Input: part model. Units: mm. Frame: model coordinates. Face numbers are marked on the shaded views. A direction names the side the tool comes from. Give positions to 0.01 mm unless a question says otherwise; leave off trailing zeros. Loops run counter-clockwise (first coordinate to the right, second up) from the corner with the lowest first, then second, coordinate; pieces in that order, holes last. Notation, with made-up numbers: (66.5, 10) - (100.5, 10) arc R20 cw to (100.5, 35) - close; hole circle Ø9 at (-12.5, 29). An arc over 180 degrees is marked (long way). One line per question, with ' | ' between items. Start each with the question number.
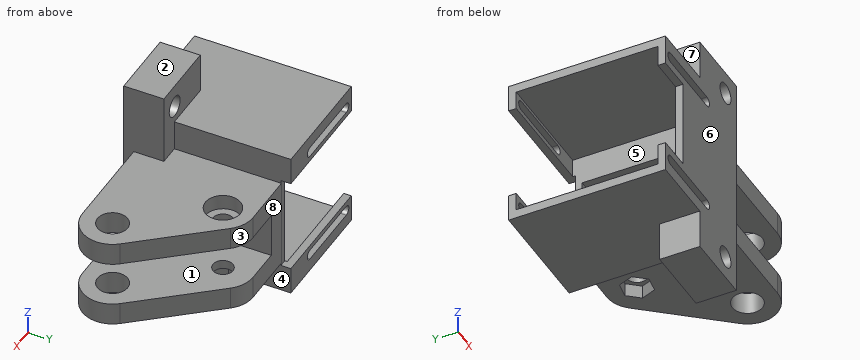
from build123d import *

# Parameters (mm, degrees)
EXTRUDE_1_DEPTH             = 9
SKETCH_2_W                  = 27.565905012
SKETCH_2_H                  = 27.320888862
CUT_EXTRUDE_1_DEPTH         = 4.5
CUT_EXTRUDE_2_DEPTH         = 2.7
SKETCH_5_R                  = 3
CUT_EXTRUDE_3_DEPTH         = 55.658762352
SKETCH_8_W                  = 23.244247806
SKETCH_8_H                  = 18
EXTRUDE_2_DEPTH             = 1.879111138
SKETCH_9_W                  = 23.244247806
SKETCH_9_H                  = 18
EXTRUDE_3_DEPTH             = 2
SKETCH_10_W                 = 23.244247806
SKETCH_10_H                 = 31.2
EXTRUDE_4_DEPTH             = 6.1
SKETCH_11_W                 = 23.244247806
SKETCH_11_H                 = 31.2
EXTRUDE_5_DEPTH             = 6.1
SHELL_START                 = -13.6
SHELL_2_OUTLINE_W           = 21.744247806
SHELL_2_OUTLINE_H           = 28.2
SHELL_2_DEPTH               = 27.2
SHELL_START_2               = -7.5
SHELL_2_2_OUTLINE_W         = 3.923676383
SHELL_2_2_OUTLINE_H         = 24.320888862
SHELL_2_2_DEPTH             = 15
SHELL_2_3_DEPTH             = 1.5
SHELL_START_3               = 6
SHELL_2_4_DEPTH             = 1.5
CUT_EXTRUDE_4_DEPTH         = 59.399058212
CUT_EXTRUDE_START           = -2
SKETCH_13_W                 = 23.244247806
SKETCH_13_H                 = 19.2
CUT_EXTRUDE_5_DEPTH         = 2
SKETCH_15_W                 = 10
SKETCH_15_H                 = 8
EXTRUDE_6_DEPTH             = 8
EXTRUDE_7_REACH             = 59.279
SKETCH_19_W                 = 4
SKETCH_19_H                 = 8
EXTRUDE_7_DIRECTION_2_REACH = 59.279
SKETCH_17_R                 = 2.1
CUT_EXTRUDE_6_DEPTH         = 61.959412727
SKETCH_20_W                 = 21.744247806
SKETCH_20_H                 = 28.2
EXTRUDE_8_DEPTH             = 0.3
SKETCH_21_W                 = 21.744247806
SKETCH_21_H                 = 28.2
EXTRUDE_9_DEPTH             = 0.3
CUT_EXTRUDE_7_REACH         = 62.959
SKETCH_22_W                 = 6.791501739
SKETCH_22_H                 = 18


# Read off the part's stored shape, not the designer's step: 抽壳2
with BuildPart() as part:
    # 草图1 → 凸台-拉伸1 (new, symmetric)
    with BuildSketch(Plane.XY):
        with BuildLine():
            Line((-8.259485535, 19.17761452), (4.596266659, 3.856725658))
            ThreePointArc((4.596266659, 3.856725658), (5.437846722, -2.53570957), (0, -6))
            Line((0, -6), (-47, -6))
            Line((-47, -6), (-47, 21.320888862))
            Line((-47, 21.320888862), (-12.855752194, 21.320888862))
            ThreePointArc((-12.855752194, 21.320888862), (-10.320042623, 20.758735585), (-8.259485535, 19.17761452))
        make_face()
    extrude(amount=EXTRUDE_1_DEPTH, both=True)

    # 草图2 → 切除-拉伸1 (cut, symmetric)
    with BuildSketch(Plane.XY):
        with Locations((-6.049123305, 7.660444431)):
            Rectangle(SKETCH_2_W, SKETCH_2_H)
    extrude(amount=CUT_EXTRUDE_1_DEPTH, both=True, mode=Mode.SUBTRACT)

    # 草图3 → 切除-旋转1 (revolve, cut)
    with BuildSketch(Plane(origin=(0, 0, 0), x_dir=(-0.642787609686538, 0.7660444431189792, 0), z_dir=(0.7660444431189791, 0.6427876096865379, 0)), mode=Mode.PRIVATE) as cut_revolve_1_sk:
        Polygon((19.999690983, -9), (17.499690983, -9), (17.499690983, -6.3), (17.999690983, -6.3), (17.999690983, 6), (16.499690983, 6), (16.499690983, 9), (19.999690983, 9), align=None)
    revolve(cut_revolve_1_sk.sketch.rotate(Axis((-12.855553561, 15.320652142, -10), (0, 0, 1)), 230), axis=Axis((-12.855553561, 15.320652142, -10), (0, 0, 1)), mode=Mode.SUBTRACT)

    # 草图4 → 切除-拉伸2 (cut)
    with BuildSketch(Plane(origin=(0, 0, -9), x_dir=(-1, 0, 0), z_dir=(0, 0, -1))):
        Polygon((11.76974521, 18.304668488), (9.728415424, 15.872322699), (10.814223775, 12.888306353), (13.941361912, 12.336635795), (15.982691699, 14.768981584), (14.896883348, 17.752997931), align=None)
    extrude(amount=-CUT_EXTRUDE_2_DEPTH, mode=Mode.SUBTRACT)

    # 草图5 → 切除-拉伸3 (cut, through all)
    with BuildSketch(Plane.XY.offset(9)):
        Circle(SKETCH_5_R)
    extrude(amount=-CUT_EXTRUDE_3_DEPTH, mode=Mode.SUBTRACT)

    # 草图8 → 凸台-拉伸2 (add)
    with BuildSketch(Plane(origin=(0, 21.320888862, 0), x_dir=(1, 0, 0), z_dir=(0, 1, 0))):
        with Locations((-35.377876097, 0)):
            Rectangle(SKETCH_8_W, SKETCH_8_H)
    extrude(amount=EXTRUDE_2_DEPTH)

    # 草图9 → 凸台-拉伸3 (add)
    with BuildSketch(Plane.XZ.offset(6)):
        with Locations((-35.377876097, 0)):
            Rectangle(SKETCH_9_W, SKETCH_9_H)
    extrude(amount=EXTRUDE_3_DEPTH)

    # 草图10 → 凸台-拉伸4 (add)
    with BuildSketch(Plane.XY.offset(9)):
        with Locations((-35.377876097, 7.6)):
            Rectangle(SKETCH_10_W, SKETCH_10_H)
    extrude(amount=EXTRUDE_4_DEPTH)

    # 草图11 → 凸台-拉伸5 (add)
    with BuildSketch(Plane(origin=(0, 0, -9), x_dir=(-1, 0, 0), z_dir=(0, 0, -1))):
        with Locations((35.377876097, 7.6)):
            Rectangle(SKETCH_11_W, SKETCH_11_H)
    extrude(amount=EXTRUDE_5_DEPTH)

    # 抽壳2 outline → 抽壳2 (cut)
    with BuildSketch(Plane.XY.offset(SHELL_START)):
        with Locations((-36.127876097, 7.6)):
            Rectangle(SHELL_2_OUTLINE_W, SHELL_2_OUTLINE_H)
    extrude(amount=SHELL_2_DEPTH, mode=Mode.SUBTRACT)

    # Shell 2 2 outline → Shell 2 2 (cut)
    with BuildSketch(Plane.XY.offset(SHELL_START_2)):
        with Locations((-23.293914003, 7.660444431)):
            Rectangle(SHELL_2_2_OUTLINE_W, SHELL_2_2_OUTLINE_H)
    extrude(amount=SHELL_2_2_DEPTH, mode=Mode.SUBTRACT)

    # Shell 2 3 outline → Shell 2 3 (cut)
    with BuildSketch(Plane.XY.offset(SHELL_START_2)):
        with BuildLine():
            Line((-9.700771165, 11.561572286), (-14.533621013, 10.708990515))
            Line((-14.533621013, 10.708990515), (-17.68840341, 14.46807037))
            Line((-17.68840341, 14.46807037), (-16.010335958, 19.079731997))
            Line((-16.010335958, 19.079731997), (-12.136777385, 19.763081477))
            ThreePointArc((-12.136777385, 19.763081477), (-12.495104697, 19.806413735), (-12.855752194, 19.820888862))
            Line((-12.855752194, 19.820888862), (-21.332075811, 19.820888862))
            Line((-21.332075811, 19.820888862), (-21.332075811, -4.5))
            Line((-21.332075811, -4.5), (0, -4.5))
            ThreePointArc((0, -4.5), (-4.078385042, 1.901782178), (3.447199994, 2.892544244))
            Line((3.447199994, 2.892544244), (-9.4085522, 18.213433106))
            ThreePointArc((-9.4085522, 18.213433106), (-9.939002288, 18.747632212), (-10.551084785, 19.18592549))
            Line((-10.551084785, 19.18592549), (-8.022703713, 16.173233913))
            Line((-8.022703713, 16.173233913), (-9.700771165, 11.561572286))
        make_face()
    extrude(amount=SHELL_2_3_DEPTH, mode=Mode.SUBTRACT)

    # Shell 2 4 outline → Shell 2 4 (cut)
    with BuildSketch(Plane.XY.offset(SHELL_START_3)):
        with BuildLine():
            Line((3.447199994, 2.892544244), (-8.007430451, 16.543641228))
            ThreePointArc((-8.007430451, 16.543641228), (-14.968890991, 10.789227983), (-15.034514198, 19.820888862))
            Line((-15.034514198, 19.820888862), (-21.332075811, 19.820888862))
            Line((-21.332075811, 19.820888862), (-21.332075811, -4.5))
            Line((-21.332075811, -4.5), (0, -4.5))
            ThreePointArc((0, -4.5), (-4.078385042, 1.901782178), (3.447199994, 2.892544244))
        make_face()
    extrude(amount=SHELL_2_4_DEPTH, mode=Mode.SUBTRACT)

    # 草图12 → 切除-拉伸4 (cut, through all)
    with BuildSketch(Plane.XZ.offset(8)):
        with BuildLine():
            Line((-45.055752194, 12.6), (-31.055752194, 12.6))
            ThreePointArc((-31.055752194, 12.6), (-30.055752194, 11.6), (-31.055752194, 10.6))
            Line((-31.055752194, 10.6), (-45.055752194, 10.6))
            ThreePointArc((-45.055752194, 10.6), (-46.055752194, 11.6), (-45.055752194, 12.6))
        make_face()
        with BuildLine():
            Line((-45.055752194, -10.6), (-31.055752194, -10.6))
            ThreePointArc((-31.055752194, -10.6), (-30.055752194, -11.6), (-31.055752194, -12.6))
            Line((-31.055752194, -12.6), (-45.055752194, -12.6))
            ThreePointArc((-45.055752194, -12.6), (-46.055752194, -11.6), (-45.055752194, -10.6))
        make_face()
    extrude(amount=-CUT_EXTRUDE_4_DEPTH, mode=Mode.SUBTRACT)

    # 草图13 → 切除-拉伸5 (cut)
    with BuildSketch(Plane(origin=(0, 23.2, 0), x_dir=(1, 0, 0), z_dir=(0, 1, 0)).offset(CUT_EXTRUDE_START)):
        with Locations((-35.377876097, 0)):
            Rectangle(SKETCH_13_W, SKETCH_13_H)
    extrude(amount=CUT_EXTRUDE_5_DEPTH, mode=Mode.SUBTRACT)

    # 草图15 → 凸台-拉伸6 (add)
    with BuildSketch(Plane.XY.offset(15.1)):
        with Locations((-28.755752194, -4)):
            Rectangle(SKETCH_15_W, SKETCH_15_H)
    extrude_6 = extrude(amount=EXTRUDE_6_DEPTH)

    # 镜向1: 凸台-拉伸6 across plane
    add(extrude_6.mirror(Plane.XY))

    # 凸台-拉伸7: up to this face of the body (flat: up to its plane)
    extrude_7_end = Plane(part.part.faces().sort_by_distance((-28.755752194, -4, 23.1))[0])
    # 草图19 → 凸台-拉伸7 (add, up to the picked face)
    with BuildSketch(Plane.XY, mode=Mode.PRIVATE) as extrude_7_sk1:
        with Locations((-21.755752194, -4)):
            Rectangle(SKETCH_19_W, SKETCH_19_H)
    extrude_7_tool1 = split(extrude(extrude_7_sk1.sketch, amount=EXTRUDE_7_REACH, mode=Mode.PRIVATE), bisect_by=extrude_7_end, keep=Keep.BOTH, mode=Mode.PRIVATE)
    add(extrude_7_tool1.solids().sort_by(Axis((-21.755752, -4, 0), (0, 0, 1)))[0])

    # 凸台-拉伸7 direction 2: up to this face of the body (flat: up to its plane)
    extrude_7_direction_2_end = Plane(part.part.faces().sort_by_distance((-28.755752194, -4, -23.1))[0])
    # 草图19 → 凸台-拉伸7 direction 2 (add, up to the picked face)
    with BuildSketch(Plane.XY, mode=Mode.PRIVATE) as extrude_7_direction_2_sk1:
        with Locations((-21.755752194, -4)):
            Rectangle(SKETCH_19_W, SKETCH_19_H)
    extrude_7_direction_2_tool1 = split(extrude(extrude_7_direction_2_sk1.sketch, amount=-EXTRUDE_7_DIRECTION_2_REACH, mode=Mode.PRIVATE), bisect_by=extrude_7_direction_2_end, keep=Keep.BOTH, mode=Mode.PRIVATE)
    add(extrude_7_direction_2_tool1.solids().sort_by(Axis((-21.755752, -4, 0), (0, 0, -1)))[0])

    # 草图17 → 切除-拉伸6 (cut, through all)
    with BuildSketch(Plane.XZ.offset(8)):
        with Locations(Location((-23.897040888, 18.5, 0), (0, 0, 270))):
            Circle(SKETCH_17_R)
        with Locations(Location((-23.897040888, -18.5, 0), (0, 0, 270))):
            Circle(SKETCH_17_R)
    extrude(amount=-CUT_EXTRUDE_6_DEPTH, mode=Mode.SUBTRACT)

    # 草图20 → 凸台-拉伸8 (add)
    with BuildSketch(Plane.XY.offset(-13.6)):
        with Locations((-36.127876097, 7.6)):
            Rectangle(SKETCH_20_W, SKETCH_20_H)
    extrude(amount=EXTRUDE_8_DEPTH)

    # 草图21 → 凸台-拉伸9 (add)
    with BuildSketch(Plane(origin=(0, 0, 13.6), x_dir=(-1, 0, 0), z_dir=(0, 0, -1))):
        with Locations((36.127876097, 7.6)):
            Rectangle(SKETCH_21_W, SKETCH_21_H)
    extrude(amount=EXTRUDE_9_DEPTH)

    # 草图22 → 切除-拉伸7 (cut, up to next)
    with BuildSketch(Plane.XZ.offset(8), mode=Mode.PRIVATE) as cut_extrude_7_sk1:
        with Locations((-43.604249131, 0)):
            Rectangle(SKETCH_22_W, SKETCH_22_H)
    cut_extrude_7_tool1 = extrude(cut_extrude_7_sk1.sketch, amount=-CUT_EXTRUDE_7_REACH, mode=Mode.PRIVATE) & part.part
    add(cut_extrude_7_tool1.solids().sort_by_distance((-43.604249, -8, 0))[0], mode=Mode.SUBTRACT)


solid = part.part
Q1. Section C-C, the plane z = -3. Output: boundary loops of the cut face in (x, y), plus the area to 3 significant figures.
Q2. Section D-D, the plane y = -2. Count the separate pieces of the cut face and the enclosed holes in it, plus the area to 3 significant figures.
Q3. Section A-A, the plane z = 18.5. Output: boundary loops of the cut face in (x, y), plus the area to 3 significant figures.
Q4. First-contact query: pin 1 (7 mm diameter, centred on x = -26, z = 19, fed in from +Y); pin 2 (0.8 mm diameter, centred on y = -7.5, z = 0, fed in from -X); pin 3 (3 mm diameter, centred on y = 17, z = 4.5, fed in from +X). Flat tips, straight axial feed; report the tip coordinate or a pass-through.
Q5. Line query: L1, parallel to Z at x = -13, y = 1.5; L2, parallel to Z at x = -17.5, y = 16; L3, parallel to Y at x = 1, z = -7. Output: solid intervals per line, ascending. Write a range as from..to.
Q6. Access query for the marked faces 4, 5, 6, 7 and 8. Directions: +Z, -Z, +X, -X, +Y, -Y. A direction counts if a zero-diameter tool reaches every point of the face in a straight line with its end or side. Return the directions, or none.
Q7. Section B-B, the plane z = -11.6. Output: boundary loops of the cut face in (x, y), plus the area to 3 significant figures.
Q8. Draft query along Z for the marked faces 1, 2 and 3. Return one class per face: +Z half, -Z half, draft (parallel to the pull), parting line (faces both ways), or undercut.
Solved:
1) outline: (-40.21, -8) - (-19.76, -8) - (-19.76, 0) - (-19.83, 0) - (-19.83, 21.32) - (-23.76, 21.32) - (-23.76, 21.2) - (-25.26, 21.2) - (-25.26, 19.82) - (-21.33, 19.82) - (-21.33, 0) - (-23.76, 0) - (-23.76, -4.5) - (-25.26, -4.5) - (-25.26, -6.5) - (-40.21, -6.5) - close | area: 97.4 mm²
2) separate pieces: 3 | enclosed holes: 4 | area: 559 mm²
3) outline: (-33.76, -8) - (-26, -8) - (-26, 0) - (-33.76, 0) - close; (-21.8, -8) - (-19.76, -8) - (-19.76, 0) - (-21.8, 0) - close | area: 78.4 mm²
4) pin 1: stops at y = 0 | pin 2: stops at x = -40.21 | pin 3: stops at x = -5.17
5) L1: z = -9..-7.5, -6..-4.5, 4.5..6, 7.5..9 | L2: z = -9..-7.5, -6..-4.5, 4.5..9 | L3: y = -5.92..-2.83, 2.83..4.39, 5.81..8.14
6) face 4: -Z, +X, +Y | face 5: -X | face 6: +Z, -Z, +X, -X, -Y | face 7: +Z, -X, +Y, -Y | face 8: +Z, -Z, +X, -X, +Y
7) outline: (-47, -8) - (-46.06, -8) - (-46.06, -6.5) - (-47, -6.5) - close; (-47, 21.7) - (-46.06, 21.7) - (-46.06, 23.2) - (-47, 23.2) - close; (-30.06, -8) - (-19.76, -8) - (-19.76, 0) - (-23.76, 0) - (-23.76, 23.2) - (-30.06, 23.2) - (-30.06, 21.7) - (-25.26, 21.7) - (-25.26, -6.5) - (-30.06, -6.5) - close | area: 96.0 mm²
8) face 1: undercut | face 2: +Z half | face 3: draft
